Design review of the part built by this model. Coordinates are the model's own, in mm. Face numbers are marked on the shaded views. A direction names the side the tool comes from. Coordinates: 2 decimals unless noted, no trailing zeros. Write each loop counter-clockwise with the first axis right and the second up, starting at its lowest first coordinate (ties: lowest second). Pieces come first, ordered by that corner, then holes. Notation, with made-up numbers: (67.25, 59) - (71.25, 59) arc R19 ccw to (71.25, 64) - close; hole circle Ø9 at (-27, 20.25). An arc over 180 degrees is marked (long way). Use a Markdown table: item, result.
from build123d import *

# Parameters (mm, degrees)
BOSS_EXTRUDE1_DEPTH = 40
CUT_EXTRUDE1_DEPTH  = 8
CUT_EXTRUDE2_DEPTH  = 134.221619867
BOSS_EXTRUDE2_START = -20
SKETCH5_R           = 19
SKETCH5_R_2         = 10
BOSS_EXTRUDE2_DEPTH = 20
SKETCH6_R           = 5
BOSS_EXTRUDE3_DEPTH = 10
SKETCH7_R           = 5
BOSS_EXTRUDE4_DEPTH = 10


with BuildPart() as part:
    # Sketch1 → Boss-Extrude1 (new body)
    with BuildSketch(Plane.XY):
        Polygon((0, 0), (20, 0), (20, 20), (56, 20), (56, 0), (76, 0), (76, 64), (82, 64), (82, 69), (76, 100), (0, 100), (-6, 69), (-6, 64), (0, 64), align=None)
    extrude(amount=BOSS_EXTRUDE1_DEPTH)

    # Sketch2 → Cut-Extrude1 (cut)
    with BuildSketch(Plane.XY.offset(40)):
        with BuildLine():
            Line((11, 100), (65, 100))
            ThreePointArc((65, 100), (38, 73), (11, 100))
        make_face()
    extrude(amount=-CUT_EXTRUDE1_DEPTH, mode=Mode.SUBTRACT)

    # Sketch4 → Cut-Extrude2 (cut, through all)
    with BuildSketch(Plane.XY.offset(32)):
        with BuildLine():
            Line((19, 100), (57, 100))
            ThreePointArc((57, 100), (38, 81), (19, 100))
        make_face()
    extrude(amount=-CUT_EXTRUDE2_DEPTH, mode=Mode.SUBTRACT)

    # Sketch5 → Boss-Extrude2 (add)
    with BuildSketch(Plane(origin=(0, 0, 0), x_dir=(-1, 0, 0), z_dir=(0, 0, -1)).offset(BOSS_EXTRUDE2_START)):
        with Locations((-38, 100)):
            Circle(SKETCH5_R)
        with Locations((-38, 100)):
            Circle(SKETCH5_R_2, mode=Mode.SUBTRACT)
    extrude(amount=BOSS_EXTRUDE2_DEPTH)

    # Sketch6 → Boss-Extrude3 (add)
    with BuildSketch(Plane.XZ.offset(-64)):
        with BuildLine():
            Line((-3.1710474, 30), (-3.1710474, 10))
            Line((-3.1710474, 10), (-25, 10))
            ThreePointArc((-25, 10), (-35, 20), (-25, 30))
            Line((-25, 30), (-3.1710474, 30))
        make_face()
        with Locations(Location((-25, 20, 0), (0, 0, 270))):
            Circle(SKETCH6_R, mode=Mode.SUBTRACT)
    extrude(amount=-BOSS_EXTRUDE3_DEPTH)

    # Sketch7 → Boss-Extrude4 (add)
    with BuildSketch(Plane.XZ.offset(-64)):
        with BuildLine():
            Line((78.953464746, 30), (78.953464746, 10))
            Line((78.953464746, 10), (101, 10))
            ThreePointArc((101, 10), (111, 20), (101, 30))
            Line((101, 30), (78.953464746, 30))
        make_face()
        with Locations(Location((101, 20, 0), (0, 0, 270))):
            Circle(SKETCH7_R, mode=Mode.SUBTRACT)
    extrude(amount=-BOSS_EXTRUDE4_DEPTH)


solid = part.part
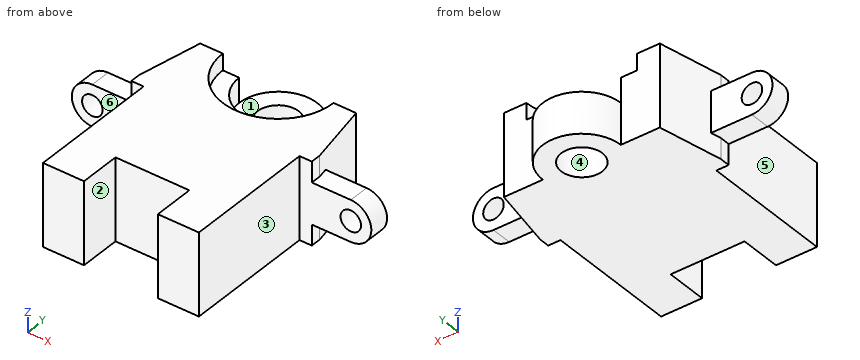
(1) Take a section at A-A on x = 38. Write out the cut boundary in (y, z).
Determined:
| item | result |
|---|---|
| outline | (20, 0) - (90, 0) - (90, 20) - (81, 20) - (81, 32) - (73, 32) - (73, 40) - (20, 40) - close; (110, 0) - (119, 0) - (119, 20) - (110, 20) - close |
(2) For L1, parallel to X at y = 69.25, z = 20; L2, parallel to X at y = 13, z = 18.5; L3, parallel to X at y = 69, z = 35, list the stretches that pass through material, from the lowest coordinate up. Write a range as from..to.
Determined:
| item | result |
|---|---|
| L1 | -35..-30, -20..96, 106..111 |
| L2 | 0..20, 56..76 |
| L3 | -6..82 |
(3) Machinability: for the marked faces 1, 2 and 3, which of the approach directions +Z, -Z, +X, -X, +Y, -Y give a long, thin tool a straight path to every point of the face, cutting with its end or side? Answer none if there is none.
Determined:
| item | result |
|---|---|
| face 1 | +Z, +Y |
| face 2 | +Z, -Z, -Y |
| face 3 | +Z, -Z, +X, -Y |
(4) Draft analysis for pull direction Y (two halves, no side actions). For the marked faces 4, 5 and 6, state which applies: +Y half, -Y half, draft (parallel to the pull), parting line (faces both ways), or undercut.
Determined:
| item | result |
|---|---|
| face 4 | undercut |
| face 5 | draft |
| face 6 | -Y half |
(5) For pin 1 (17.5 mm diameter, centred on x = -13.5, z = 26, fed in from -Y); pin 2 (5 mm diameter, centred on x = 77, y = 57.5, fed in from -Z); pin 3 (9 mm diameter, centred on x = -25, z = 20, fed in from -Y); pin 4 (11.5 mm diameter, centred on x = 32.5, y = 93.5, fed in from +Z), all flat-tipped, find the tip position at first contact; note any pin that passes through.
Determined:
| item | result |
|---|---|
| pin 1 | y = 64 |
| pin 2 | z = 0 |
| pin 3 | through |
| pin 4 | z = 20 |
(6) Take a section at D-D on x = 79. Write out the cut boundary in (y, z), and give its area (3 significant figures).
Determined:
| item | result |
|---|---|
| outline | (64, 0) - (84.5, 0) - (84.5, 40) - (64, 40) - close |
| area | 820 mm2 |
(7) Take a section at C-C on x = 4. Write out the cut boundary in (y, z), and give its area (3 significant figures).
Determined:
| item | result |
|---|---|
| outline | (0, 0) - (100, 0) - (100, 40) - (0, 40) - close |
| area | 4,000 mm2 |
(8) Take a section at B-B on z = 37.5. Write out the cut boundary in (x, y).
Determined:
| item | result |
|---|---|
| outline | (-6, 64) - (0, 64) - (0, 0) - (20, 0) - (20, 20) - (56, 20) - (56, 0) - (76, 0) - (76, 64) - (82, 64) - (82, 69) - (76, 100) - (65, 100) arc R27 cw to (11, 100) - (0, 100) - (-6, 69) - close |
